Can you work these out from the model? Positions are in its coordinate system, mm. Face numbers are marked on the shaded views. A direction names the side the tool comes from. Give positions to 0.01 mm unless a question says otherwise; leave off trailing zeros. Order: outer loops, then holes, each group sorted by start corner. A loop starts at its lowest first (then second) coordinate and runs counter-clockwise, first axis right, second up. Notation, with made-up numbers: (-30.5, 56) - (-3.5, 56) arc R29 cw to (-3.5, 82) - close; hole circle Ø11 at (56, -25.75). An arc over 180 degrees is marked (long way). Return JSON: item names as keys, results as strings.
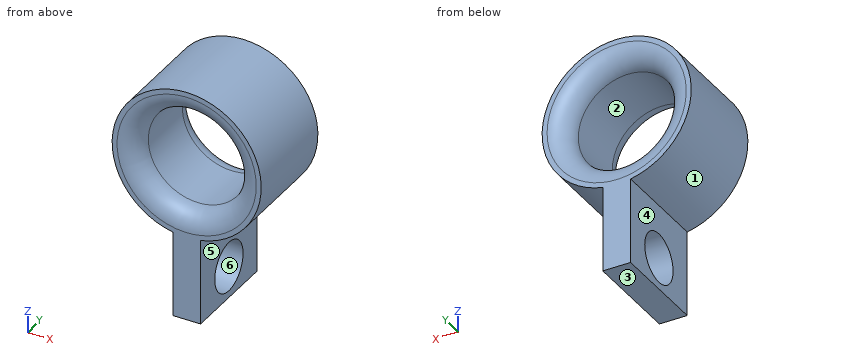
```python
from build123d import *

# Parameters (mm, degrees)
F0_R     = 4.7625
F0_R_2   = 3.175
F1_DEPTH = 3.175
F2_W     = 6.35
F2_H     = 6.35
F2_R     = 1.5875
F3_DEPTH = 0.889
F4_R     = 1.27


with BuildPart() as f1:
    # F0 (on Front) → F1 (new body, symmetric)
    with BuildSketch(Plane.XZ):
        Circle(F0_R)
        Circle(F0_R_2, mode=Mode.SUBTRACT)
    extrude(amount=F1_DEPTH, both=True)

    # F2 (on Right) → F3 (join, symmetric)
    with BuildSketch(Plane.YZ):
        with Locations((0, -6.985)):
            Rectangle(F2_W, F2_H)
        with Locations((0, -8.128)):
            Circle(F2_R, mode=Mode.SUBTRACT)
    extrude(amount=F3_DEPTH, both=True)

    # F4
    f4_edges = [f1.edges().sort_by_distance(p)[0] for p in [
        (-3.175, -3.175, 0),
        (-3.175, 3.175, 0),
    ]]
    fillet(f4_edges, radius=F4_R)


solid = f1.part
```
1. For pin 1 Ø3 at (y, z) = (0.5, -8) entering from -X; pin 2 Ø3 at (x, y) = (-2.5, -0.5) entering from -Z, each with a flat end and sliding along its axis, tell me the tip position at first contact or that it passes through.
Checks:
{"pin 1": "x = -0.89", "pin 2": "z = -4.66"}
2. On a 3-axis mill with a long thin cutter (end or side, diameter ignored), from which of +Z, -Z, +X, -X, +Y, -Y can I reach the whole of each face in a straight line? I mean the marked faces 5 and 6. Say none if no direction works.
Checks:
{"face 5": "-Z, +X, +Y, -Y", "face 6": "+X, -X"}
3. Suppose I cut it at B-B (z = -7). List the corners of the cut face in (x, y) for me (3 decimals).
Checks:
{"outline": "(-0.889, -3.175) - (0.889, -3.175) - (0.889, -1.117) - (-0.889, -1.117) - close; (-0.889, 1.117) - (0.889, 1.117) - (0.889, 3.175) - (-0.889, 3.175) - close"}
4. If I drill on L1, parallel to Z at x = 0.75, y = -0.75; L2, parallel to X at y = 1, z = -5.5; L3, parallel to Z at x = -0.75, y = -0.5, over which ranges is the centre line in solid material (lowest first)? Write a range as [from, to].
Checks:
{"L1": "[-10.16, -9.53], [-6.73, -3.09], [3.09, 4.7]", "L2": "[-0.89, 0.89]", "L3": "[-10.16, -9.63], [-6.62, -3.09], [3.09, 4.7]"}
5. Suppose I cut it at A-A (y = 0). State how many separate pieces and enclosed holes the cut face has, plus the area to 3 significant figures.
Checks:
{"separate pieces": "2", "enclosed holes": "1", "area": "43.6 mm^2"}
6. Suppose I cut it at D-D (y = -2.5). List the corners of the cut face in (x, z) for me (1 decimal).
Checks:
{"outline": "(-0.9, -10.2) - (0.9, -10.2) - (0.9, -4.7) arc R4.8 ccw (long way) to (-0.9, -4.7) - close; hole circle Ø6.6 at (0, 0)"}
7. Thinking about a two-plate mould opening in X: for the marked faces 1, 2, 3 and 4, which applies, +X half, -X half, draft (parallel to the pull), parting line (faces both ways), or undercut?
Checks:
{"face 1": "parting line", "face 2": "undercut", "face 3": "draft", "face 4": "-X half"}
